Autodesk Inventor part; units mm, degrees
ref_plane "YZ Plane" through (0, 0, 0) normal (1, 0, 0) x (0, 1, 0)
ref_plane "XZ Plane" through (0, 0, 0) normal (0, 1, 0) x (-1, 0, 0)
ref_plane "XY Plane" through (0, 0, 0) normal (0, 0, 1) x (1, 0, 0)
sketch "Sketch3" plane through (0, 0, 0) normal (0, 0, 1) x (1, 0, 0)
  line L0 (0, 0) -> (570, 0)
  line L1 (570, 0) -> (570, 35)
  line L2 (570, 35) -> (0, 35)
  line L3 (0, 35) -> (0, 0)
  dimension "d3" = 570
  dimension "d4" = 35
extrude "Extrusion2" add sketch "Sketch3" along normal blind 25
sketch "Sketch4" plane through (0, 0, 25) normal (0, 0, 1) x (1, 0, 0)
  point P0 (0, 0)
sketch "Sketch5" plane through (0, 0, 25) normal (0, 0, 1) x (1, 0, 0)
  line L0 (0, 35) -> (0, 0)
  point P0 (20, 17.5)
hole "Hole1" at (20, 17.5, 25) direction (0, 0, -1) diameter 22 end through all
fillet "Fillet4" radius 17.5 1 edges at (0, 35, 12.5)
fillet "Fillet5" radius 17.5 1 edges at (0, 0, 12.5)
properties part number "RoboArm 2020 Arm"
Build history of the part. All positions in model axes, mm. Coordinates: 2 decimals unless noted, no trailing zeros. One line per question, with ' | ' between items. Start each with the question number.
Q1. Two-plate mould, pull along X, no slides. Class faces 1 (the face through (570, 17, 12)), 2 (the face through (5.26, 30.01, 12.68)), 3 (the face through (281, 18, 25)), 4 (the face through (29.759, 12.424, 12.325)): +X half, -X half, draft (parallel to the pull), parting line (faces both ways), or undercut.
Q2. Flat gauge pins, fed straight in: pin 1 Ø4 at (y, z) = (13, 3.5) entering from -X; pin 2 Ø2 at (y, z) = (10, 16.5) entering from -X. Where does each tip first touch, or does it go through?
Q3. Probe L1, parallel to Y at x = 20, z = 19; L2, parallel to X at y = 16, z = 1.75; L3, parallel to X at y = 17.5, z = 19.5. List the from-to ranges inside material, lowest first. Write a range as from..to.
Check values:
1) face 1: +X half | face 2: -X half | face 3: draft | face 4: undercut
2) pin 1: stops at x = 0.18 | pin 2: stops at x = 1.25
3) L1: y = 0..6.5, 28.5..35 | L2: x = 0.06..9.1, 30.9..570 | L3: x = 0..9, 31..570
